from build123d import *

# Parameters (mm, degrees)
FASE1_SIZE = 0.5


with BuildPart() as part:
    # Skizze1 → Rotation1 (revolve)
    with BuildSketch(Plane.XY, mode=Mode.PRIVATE) as rotation1_sk:
        Polygon((5, 5.5), (5, 14.5), (4, 14.5), (4, 15.6), (5, 15.6), (5, 20), (0, 20), (0, 0), (5, 0), (5, 4.4), (4, 4.4), (4, 5.5), align=None)
    revolve(rotation1_sk.sketch.rotate(Axis((0, 0, 0), (0, 1, 0)), 90), axis=Axis((0, 0, 0), (0, 1, 0)))

    # Fase1
    fase1_edges = [part.edges().sort_by_distance(p)[0] for p in [
        (0, 20, 5),
        (0, 0, 5),
    ]]
    chamfer(fase1_edges, length=FASE1_SIZE)


solid = part.part
CAD build for the part. Positions are in the model's coordinates, mm. A direction names the side the tool comes from. Round coordinates to 2 decimals unless told otherwise and drop trailing zeros. Order: outer loops, then holes, each group sorted by start corner. A loop starts at its lowest first (then second) coordinate and runs counter-clockwise, first axis right, second up. Notation, with made-up numbers: (-24, 77.5) - (31, 77.5) arc R21 cw to (31, 86.5) - close; hole circle Ø8 at (88.25, 25.5). An arc over 180 degrees is marked (long way). Return JSON: item names as keys, results as strings.
(1) Pull direction Y, two halves, no side cores. Call faces 1 (the face through (0, 2, 5)), 2 (the face through (0, 20, 0)), 3 (the face through (3.905, 15.058, 0.867)): +Y half, -Y half, draft (parallel to the pull), parting line (faces both ways), or undercut.
Answer key:
{"face 1": "draft", "face 2": "+Y half", "face 3": "undercut"}
(2) Cut at A-A (z = 0). Give the cut face in (x, y), then the cut area to 3 significant figures.
Answer key:
{"outline": "(-5, 0.5) - (-4.5, 0) - (4.5, 0) - (5, 0.5) - (5, 4.4) - (4, 4.4) - (4, 5.5) - (5, 5.5) - (5, 14.5) - (4, 14.5) - (4, 15.6) - (5, 15.6) - (5, 19.5) - (4.5, 20) - (-4.5, 20) - (-5, 19.5) - (-5, 15.6) - (-4, 15.6) - (-4, 14.5) - (-5, 14.5) - (-5, 5.5) - (-4, 5.5) - (-4, 4.4) - (-5, 4.4) - close", "area": "195 mm^2"}
(3) Cut at B-B (x = 0). Give the cut face in (y, z).
Answer key:
{"outline": "(0, -4.5) - (0.5, -5) - (4.4, -5) - (4.4, -4) - (5.5, -4) - (5.5, -5) - (14.5, -5) - (14.5, -4) - (15.6, -4) - (15.6, -5) - (19.5, -5) - (20, -4.5) - (20, 4.5) - (19.5, 5) - (15.6, 5) - (15.6, 4) - (14.5, 4) - (14.5, 5) - (5.5, 5) - (5.5, 4) - (4.4, 4) - (4.4, 5) - (0.5, 5) - (0, 4.5) - close"}
(4) Cut at C-C (y = 1.5). Give the cut face in (x, z).
Answer key:
{"outline": "circle Ø10 at (0, 0)"}
(5) Wall check: probe 1 along Y at (x, z) = (4, 2); probe 2 along Y at (x, z) = (-1.25, 4.5); probe 3 along Z at (x, y) = (3, 2). Give the ranges that are in metal, low to high. Write a range as from..to.
Answer key:
{"probe 1": "y = 0..4.4, 5.5..14.5, 15.6..20", "probe 2": "y = 0.17..4.4, 5.5..14.5, 15.6..19.83", "probe 3": "z = -4..4"}
(6) Pin check, flat tips, straight feed: pin 1 Ø3 at (x, z) = (-2.5, -0.5) entering from -Y; pin 2 Ø2 at (y, z) = (13, -1.5) entering from -X; pin 3 Ø1.5 at (x, y) = (2, 8) entering from +Z; pin 4 Ø1.5 at (x, y) = (2, 3.5) entering from -Z. Stop position of each tip, or through.
Answer key:
{"pin 1": "stops at y = 0", "pin 2": "stops at x = -4.97", "pin 3": "stops at z = 4.84", "pin 4": "stops at z = -4.84"}
(7) Tool access for faces 4 (the face through (0, 10, 5)), 5 (the face through (3.905, 4.958, 0.867)): list every direction of +Z, -Z, +X, -X, +Y, -Y with a clear straight run to the whole face (end or side of a thin tool).
Answer key:
{"face 4": "+Y, -Y", "face 5": "none"}
(8) Cut at D-D (z = 4.25). State how many separate pieces and enclosed holes the cut face has, then the cut area to 3 significant figures.
Answer key:
{"separate pieces": "3", "enclosed holes": "0", "area": "92.7 mm^2"}
